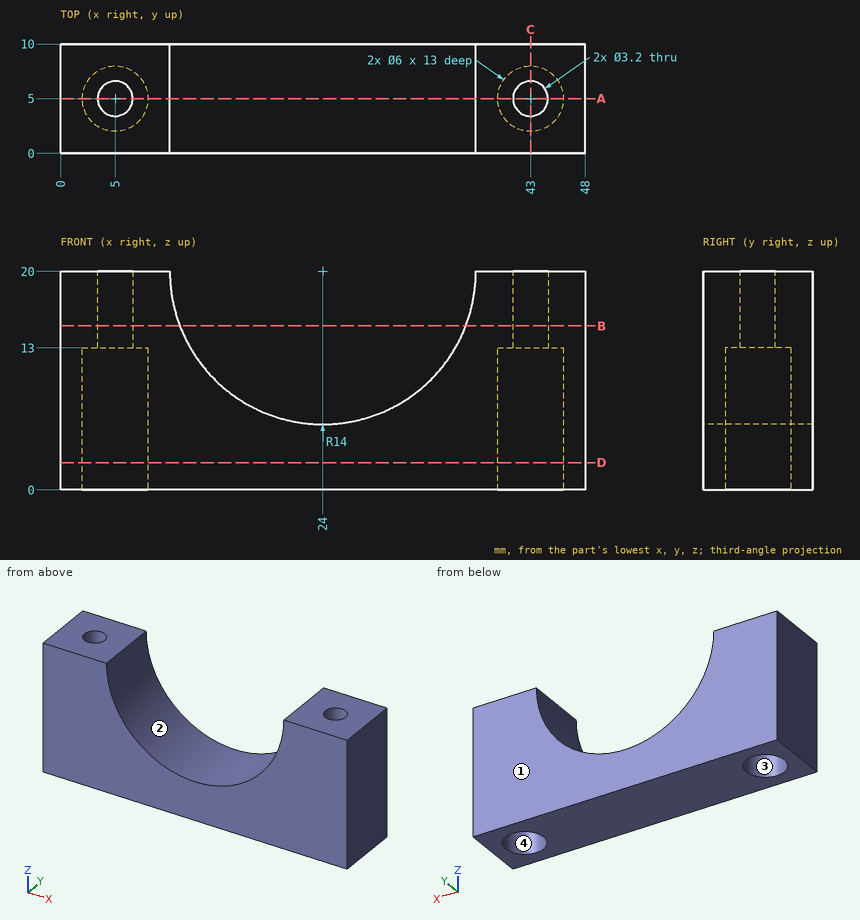
Here's the drawing with two shaded views (mm, measured from the low corner). I have some questions. Coordinates: 2 decimals unless noted, no trailing zeros. Order: outer loops, then holes, each group sorted by start corner. A loop starts at its lowest first (then second) coordinate and runs counter-clockwise, first axis right, second up.
Item 1: If we section it at D-D on z = 2.5: List the corners of the cut face in (x, y) for me, plus the area to 3 significant figures.
Result sheet:
outline: (0, 0) - (48, 0) - (48, 10) - (0, 10) - close; hole circle Ø6 at (5, 5); hole circle Ø6 at (43, 5)
area: 423 mm2
Item 2: I need wall thicknesses on line 1 (Y direction, x = 5, z = 8.75); line 2 (X direction, y = 6, z = 2); line 3 (X direction, y = 6.25, z = 4). Which ranges of each line are inside material? Lowest first, please.
Result sheet:
line 1: y = 0 to 2, 8 to 10
line 2: x = 0 to 2.17, 7.83 to 40.17, 45.83 to 48
line 3: x = 0 to 2.27, 7.73 to 40.27, 45.73 to 48
Item 3: For P1, Ø2, axis at x = 26, y = 4, coming from the -Z side; P2, Ø2.5, axis at x = 43, y = 5, coming from the +Z side; P3, Ø3, axis at x = 14, y = 4.5, coming from the +Z side, each with a flat end and sliding along its axis, tell me the tip position at first contact or that it passes through.
Result sheet:
P1: stops at z = 0
P2: passes through
P3: stops at z = 12.02
Item 4: If we section it at B-B on z = 15: List the corners of the cut face in (x, y) for me, plus the area to 3 significant figures.
Result sheet:
outline: (0, 0) - (10.92, 0) - (10.92, 10) - (0, 10) - close; (37.08, 0) - (48, 0) - (48, 10) - (37.08, 10) - close; hole circle Ø3.2 at (5, 5); hole circle Ø3.2 at (43, 5)
area: 202 mm2
Item 5: If we mould it in two halves opening along Y, with no side actions, what happens to the marked faces 1, 2, 3 and 4? For each: +Y half, -Y half, draft (parallel to the pull), parting line (faces both ways), or undercut.
Result sheet:
face 1: +Y half
face 2: draft
face 3: undercut
face 4: undercut
Item 6: If we section it at A-A on y = 5: List the corners of the cut face in (x, z) for me, plus the area to 3 significant figures.
Result sheet:
outline: (0, 0) - (2, 0) - (2, 13) - (3.4, 13) - (3.4, 20) - (0, 20) - close; (6.6, 13) - (8, 13) - (8, 0) - (40, 0) - (40, 13) - (41.4, 13) - (41.4, 20) - (38, 20) arc R14 cw to (10, 20) - (6.6, 20) - close; (44.6, 13) - (46, 13) - (46, 0) - (48, 0) - (48, 20) - (44.6, 20) - close
area: 451 mm2
Item 7: If we section it at C-C on x = 43: List the corners of the cut face in (y, z) for me, plus the area to 3 significant figures.
Result sheet:
outline: (0, 0) - (2, 0) - (2, 13) - (3.4, 13) - (3.4, 20) - (0, 20) - close; (6.6, 13) - (8, 13) - (8, 0) - (10, 0) - (10, 20) - (6.6, 20) - close
area: 99.6 mm2
